Part print with two shaded views. Sizes in mm from the minimum x, y, z corner. A direction names the side the tool comes from. Round coordinates to 2 decimals unless told otherwise and drop trailing zeros. Write each loop counter-clockwise with the first axis right and the second up, starting at its lowest first coordinate (ties: lowest second). Pieces come first, ordered by that corner, then holes. Notation, with made-up numbers: (9.25, 7.5) -> (56.25, 7.5) arc R29 ccw to (56.25, 32.5) -> close; hole circle Ø3 at (88, 61). An arc over 180 degrees is marked (long way). Answer as CSV lines item,"result".
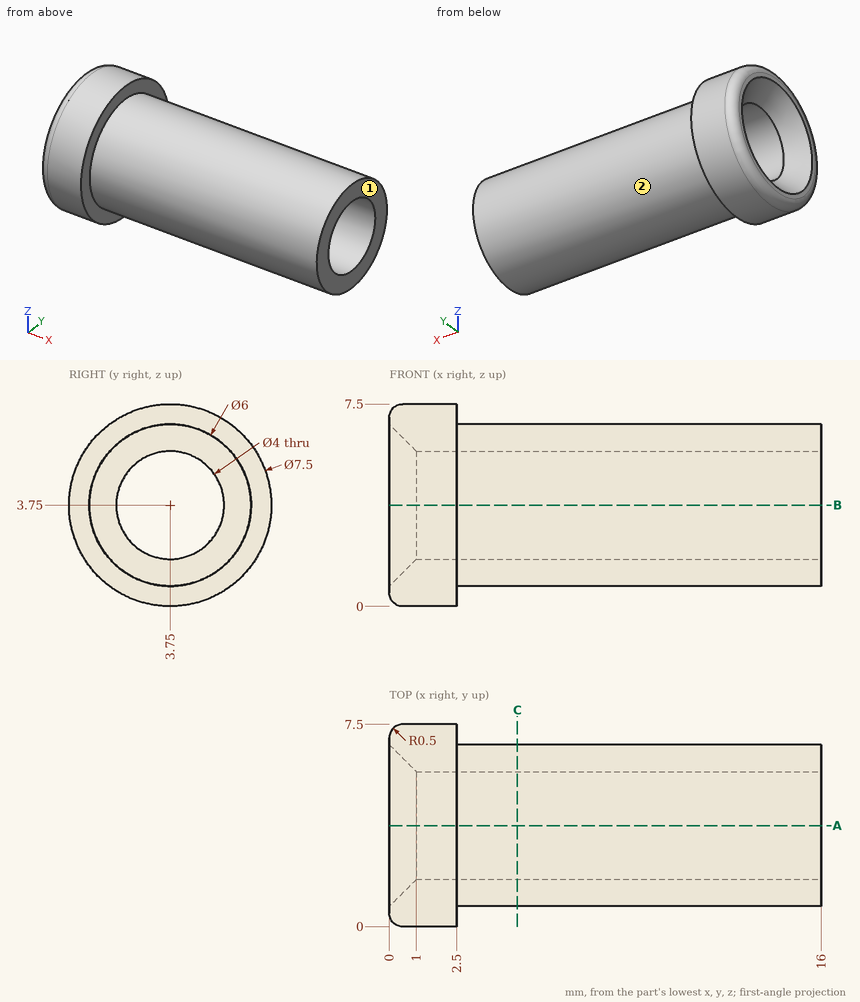
1. Drop flat-ended pins along their axis: pin 1 Ø4 at (x, y) = (2, 6.5) entering from +Z; pin 2 Ø3 at (x, z) = (6.5, 6) entering from -Y; pin 3 Ø3 at (y, z) = (3.75, 3.75) entering from +X; pin 4 Ø1.5 at (x, y) = (10.5, 4) entering from -Z. Give the stop position or say it passes through.
Results found:
pin 1,"stops at z = 7.42"
pin 2,"stops at y = 0.85"
pin 3,"passes through"
pin 4,"stops at z = 0.75"
2. Cut at C-C, the plane x = 4.75. Write the cut outline in (y, z), then the cut area to 3 significant figures.
Results found:
outline,"circle Ø6 at (3.75, 3.75); hole circle Ø4 at (3.75, 3.75)"
area,"15.7 mm2"
3. Probe line 1 along Y through (x, z) = (4.5, 3.75); line 2 along Z through (x, y) = (10, 4); line 3 along Y through (x, z) = (9.5, 2.25). List the from-to ranges inside material, lowest first.
Results found:
line 1,"y = 0.75 to 1.75, 5.75 to 6.75"
line 2,"z = 0.76 to 1.77, 5.73 to 6.74"
line 3,"y = 1.15 to 2.43, 5.07 to 6.35"
4. Which spindle directions (+Z, -Z, +X, -X, +Y, -Y) get a long thin tool onto all of the face, cutting with end or side? Do the marked faces 1 and 2. Say none if no direction does.
Results found:
face 1,"+Z, -Z, +X, +Y, -Y"
face 2,"+X"
5. Cut at A-A, the plane y = 3.75. Write the cut outline in (x, z).
Results found:
outline,"(0, 0.5) arc R0.5 ccw to (0.5, 0) -> (2.5, 0) -> (2.5, 0.75) -> (16, 0.75) -> (16, 1.75) -> (1, 1.75) -> (0, 0.75) -> close; (0, 6.75) -> (1, 5.75) -> (16, 5.75) -> (16, 6.75) -> (2.5, 6.75) -> (2.5, 7.5) -> (0.5, 7.5) arc R0.5 ccw to (0, 7) -> close"
